Geometry check sheet. Reference: the model listing, model coordinates, mm. A direction names the side the tool comes from. Give positions to 0.01 mm unless a question says otherwise; leave off trailing zeros. Loops run counter-clockwise (first coordinate to the right, second up) from the corner with the lowest first, then second, coordinate; pieces in that order, holes last.
```python
from build123d import *

# Parameters (mm, degrees)
CHAMFER1_SIZE                = 1
F_10_2_10_2_DIAMETER_HOLE1_D = 10.2


with BuildPart() as part:
    # Sketch1 → Revolve1 (revolve)
    with BuildSketch(Plane.XY, mode=Mode.PRIVATE) as revolve1_sk:
        Polygon((0, 0), (16, 0), (16, -45), (10, -45), (10, -68), (0, -68), align=None)
    revolve(revolve1_sk.sketch.rotate(Axis((0, -73, 0), (0, 1, 0)), 90), axis=Axis((0, -73, 0), (0, 1, 0)))

    # Chamfer1
    chamfer1_edges = [part.edges().sort_by_distance(p)[0] for p in [
        (0, -68, 10),
        (0, -45, 16),
        (0, 0, 16),
    ]]
    chamfer(chamfer1_edges, length=CHAMFER1_SIZE)

    # Ø10.2 (10.2) Diameter Hole1 (through all)
    with Locations(Plane(origin=(0, 0, 0), x_dir=(1, 0, 0), z_dir=(0, 1, 0))):
        with Locations((0, 0)):
            Hole(F_10_2_10_2_DIAMETER_HOLE1_D / 2)


solid = part.part
```
1) Sectioned sample at C-C on y = -59. Enter the section's corners in (x, z).
2) Depth check by flat-ended pin: P1, Ø4, axis at x = -8, y = -59, coming from the +Z side; P2, Ø2, axis at y = -15.5, z = 7, coming from the +X side; P3, Ø10, axis at y = -43, z = -8.5, coming from the -X side; P4, Ø3, axis at x = 4, z = -3, coming from the +Y side. Enter the tip coordinate at first touch or a pass-through.
3) Tool access check on faces 1 (the cylindrical face through (0, -56, 10)), 2 (the flat face through (4, -68, -4)). Record the directions out of +Z, -Z, +X, -X, +Y, -Y that give a thin tool (end or side, any length) a straight path to the whole face; none if there is none.
4) Sectioned sample at A-A on z = 0. Enter the section's corners in (x, y), plus the area to 3 significant figures.
5) Sectioned sample at B-B on y = -31.5. Enter the section's corners in (x, z), plus the area to 3 significant figures.
6) Scan lines: line 1 along Y through (x, z) = (13, -1.5); line 2 along X through (y, z) = (-10.5, 3); line 3 along Z through (x, y) = (2, -24.5). Record each from-to range of solid material in increasing order.
7) Mould release check, pull along Z, two halves, no side actions. Record for faces 3 (the cylindrical face through (-2.4, -34.5, 4.5)), 4 (the cylindrical face through (15.62, -22.8, 3.47)), 5 (the flat face through (0, 0, 6)): +Z half, -Z half, draft (parallel to the pull), parting line (faces both ways), or undercut.
Determined:
1. outline: circle Ø20 at (0, 0); hole circle Ø10.2 at (0, 0)
2. P1: stops at z = 8
2. P2: stops at x = 14.83
2. P3: stops at x = -15.61
2. P4: stops at y = 0
3. face 1: -Y
3. face 2: +Z, -Z, +X, -X, -Y
4. outline: (-16, -44) - (-15, -45) - (-10, -45) - (-10, -67) - (-9, -68) - (-5.1, -68) - (-5.1, 0) - (-15, 0) - (-16, -1) - close; (5.1, -68) - (9, -68) - (10, -67) - (10, -45) - (15, -45) - (16, -44) - (16, -1) - (15, 0) - (5.1, 0) - close
4. area: 1,200 mm2
5. outline: circle Ø32 at (0, 0); hole circle Ø10.2 at (0, 0)
5. area: 723 mm2
6. line 1: y = -45 to 0
6. line 2: x = -15.72 to -4.12, 4.12 to 15.72
6. line 3: z = -15.87 to -4.69, 4.69 to 15.87
7. face 3: undercut
7. face 4: parting line
7. face 5: draft
